Autodesk Fusion 360 part; units mm, degrees
sketch "Sketch5" plane through (0, 0, 0) normal (0, 0, 1) x (1, 0, 0)
  line L0 (3.81, -34.29) -> (-3.81, -34.29)
  line L1 (-3.81, -34.29) -> (-3.81, 34.29)
  line L2 (-3.81, 34.29) -> (3.81, 34.29)
  line L3 (3.81, 34.29) -> (3.81, -34.29)
  line L4 (3.81, -34.29) -> (-3.81, 34.29) construction
  line L5 (-3.81, -34.29) -> (3.81, 34.29) construction
  dimension "d45" = 7.62
  dimension "d46" = 68.58
extrude "Extrude3" add sketch "Sketch5" along normal blind 2.54
fillet "Fillet2" radius 3.81 4 edges at (3.81, 34.29, 1.27) (3.81, -34.29, 1.27) (-3.81, 34.29, 1.27) (-3.81, -34.29, 1.27)
sketch "Sketch6" plane through (0, 0, 2.54) normal (0, 0, 1) x (1, 0, 0)
  arc A0 (-3.81, -30.48) -> (3.81, -30.48) centre (0, -30.48) ccw
  line L0 (3.81, -30.48) -> (3.81, 30.48)
  arc A1 (3.81, 30.48) -> (-3.81, 30.48) centre (0, 30.48) ccw
  line L1 (-3.81, 30.48) -> (-3.81, -30.48)
  circle A2 centre (-0.0028, 27.94) radius 1.905
  circle A3 centre (0.0507, 10.16) radius 1.905
  circle A4 centre (0.1601, -10.16) radius 1.905
  circle A5 centre (0.0346, -27.94) radius 1.905
  point P0 (0.0507, 10.16)
  point P1 (-0.0028, 27.94)
  point P2 (0.1601, -10.16)
  point P3 (0.0346, -27.94)
  dimension "d54" = 10.16
  dimension "d55" = 27.94
  dimension "d56" = 10.16
  dimension "d57" = 27.94
  dimension "d58" = 3.81
  dimension "d59" = 3.81
  dimension "d60" = 3.81
  dimension "d61" = 3.81
extrude "Extrude4" add sketch "Sketch6" along normal blind 5.08 contours A2 | A3 | A4 | A5
equation "shelfThickness = 0.1 in"
equation "shelfWidth = 1.5 in"
equation "shelfDepth = 1.5 in"
equation "trussThickness = 0.1 in"
equation "tabInset = trussThickness / 2"
equation "tabWidth = 0.5 in"
equation "tab1Offset = tabBaseOffset + tabWidth / 2"
equation "tab2Offset = tabBaseOffset + ( tabWidth / 2 ) + tabSeparation"
equation "tabBaseOffset = 0.15 in"
equation "tabSeparation = tabWidth + 0.2 in"
equation "trussWidth = 0.3 in"
equation "trussLength = ( 2 * tab2Offset + 0.5 in )"
equation "d45 = trussWidth"
equation "d46 = trussLength"
equation "d47 = trussThickness"
equation "tabHeight = 0.3 in"
equation "studLength = 0.2 in"
equation "studDiameter = 0.15 in"
equation "d54 = tab1Offset"
equation "d55 = tab2Offset"
equation "d56 = tab1Offset"
equation "d57 = tab2Offset"
equation "d58 = studDiameter"
equation "d59 = studDiameter"
equation "d60 = studDiameter"
equation "d61 = studDiameter"
equation "d62 = studLength"
Geometry: final body of the model. Coordinates: model frame, mm. A direction names the side the tool comes from. Give positions to 0.01 mm unless a question says otherwise; leave off trailing zeros. Order: outer loops, then holes, each group sorted by start corner. A loop starts at its lowest first (then second) coordinate and runs counter-clockwise, first axis right, second up. Notation, with made-up numbers: (8.25, 71.25) -> (44.25, 71.25) arc R19 ccw to (44.25, 107.25) -> close; hole circle Ø11 at (19.25, 85). An arc over 180 degrees is marked (long way). Write each question's results on one line, items separated by ' | '. Start each with the question number.
1) Line query: line 1 (Y direction, x = 0.5, z = 3); line 2 (Z direction, x = 1.5, y = -30.5); line 3 (Y direction, x = 0.25, z = 7). Output: solid intervals per line, ascending. Write a range as from..to.
2) Set-up query: faces 5 (the flat face through (0, -28, 7.62)), 6 (the cylindrical face through (1.18, -11.77, 5.04)). Return all of +Z, -Z, +X, -X, +Y, -Y with unobstructed straight access to the full face (end or side cutting, diameter ignored); none if empty.
3) Section B-B (y = 27.94). Return loops of the section in (x, z), then the cut area to 3 significant figures.
4) Section D-D (z = 5.5). Return loops of the section in (x, y) (3 decimals).
5) Section C-C (x = 0.75). Return loops of the section in (y, z).
6) Draft query along Y for faces 1 (the cylindrical face through (2.724, 33.145, 1.288)), 2 (the cylindrical face through (-2.724, -33.145, 1.288)), 3 (the flat face through (0, -10, 7.62)), 4 (the cylindrical face through (-0.21, -29.83, 5.04)). Return one class per face: pulls with the +Y half, pulls with the -Y half, needs draft (parallel to the pull), parting line crosses it, or undercut.
7) First-contact query: pin 1 (2.5 mm diameter, centred on x = -0.5, y = 6, fed in from +Z). Flat tip, straight axial feed; report the tip coordinate or a pass-through.
Calculated:
1) line 1: -29.79..-26.09, -12.03..-8.29, 8.31..12.01, 26.1..29.78 | line 2: 0..2.54 | line 3: -29.83..-26.05, -12.06..-8.26, 8.27..12.05, 26.05..29.83
2) face 5: +Z, +X, -X, +Y, -Y | face 6: +Z
3) outline: (-3.81, 0) -> (3.81, 0) -> (3.81, 2.54) -> (1.9, 2.54) -> (1.9, 7.62) -> (-1.91, 7.62) -> (-1.91, 2.54) -> (-3.81, 2.54) -> close | area: 38.7 mm2
4) outline: circle Ø3.81 at (-0.003, 27.94); circle Ø3.81 at (0.035, -27.94); circle Ø3.81 at (0.051, 10.16); circle Ø3.81 at (0.16, -10.16)
5) outline: (-34.22, 0) -> (34.22, 0) -> (34.22, 2.54) -> (29.69, 2.54) -> (29.69, 7.62) -> (26.19, 7.62) -> (26.19, 2.54) -> (11.93, 2.54) -> (11.93, 7.62) -> (8.39, 7.62) -> (8.39, 2.54) -> (-8.35, 2.54) -> (-8.35, 7.62) -> (-11.97, 7.62) -> (-11.97, 2.54) -> (-26.17, 2.54) -> (-26.17, 7.62) -> (-29.71, 7.62) -> (-29.71, 2.54) -> (-34.22, 2.54) -> close
6) face 1: pulls with the +Y half | face 2: pulls with the -Y half | face 3: needs draft | face 4: undercut
7) pin 1: z = 2.54
